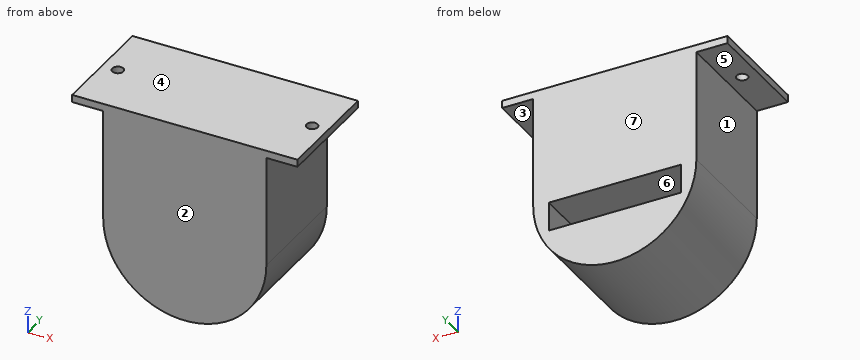
Autodesk Inventor part; units mm, degrees
ref_plane "YZ Plane" through (0, 0, 0) normal (1, 0, 0) x (0, 1, 0)
ref_plane "XZ Plane" through (0, 0, 0) normal (0, 1, 0) x (-1, 0, 0)
ref_plane "XY Plane" through (0, 0, 0) normal (0, 0, 1) x (1, 0, 0)
sketch "Sketch1" plane through (0, 0, 0) normal (0, 1, 0) x (-1, 0, 0)
  line L0 (-22, -14.1429) -> (-22, 15.8571)
  line L1 (-20.3963, 17.8571) -> (20.3963, 17.8571)
  line L2 (22, 15.8571) -> (22, -14.1429)
  arc A0 (-22, -14.1429) -> (22, -14.1429) centre (0, -14.1429) ccw
  line L3 (20.3963, 17.8571) -> (30.3963, 17.8571)
  line L4 (30.3963, 17.8571) -> (30.3963, 15.8571)
  line L5 (30.3963, 15.8571) -> (22, 15.8571)
  line L6 (-20.3963, 17.8571) -> (-30.3963, 17.8571)
  line L7 (-30.3963, 17.8571) -> (-30.3963, 15.8571)
  line L8 (-30.3963, 15.8571) -> (-22, 15.8571)
  point P0 (0, 0)
  point P1 (0, 17.8571)
  point P2 (22, 0)
  dimension "d1" = 2
  dimension "d2" = 2
  dimension "d3" = 10
  dimension "d4" = 10
  dimension "d5" = 30
  dimension "d6" = 22
extrude "Extrusion1" add sketch "Sketch1" along normal mid plane 30
sketch "Sketch2" plane through (0, 15, 0) normal (0, 1, 0) x (1, 0, 0)
  arc A0 (22, 14.1429) -> (-22, 14.1429) centre (0, 14.1429) ccw
  line L0 (-17.8, 22.1429) -> (17.8, 22.1429)
  line L1 (17.8, 22.1429) -> (17.8, 14.3429)
  line L2 (17.8, 14.3429) -> (-17.8, 14.3429)
  line L3 (-17.8, 14.3429) -> (-17.8, 22.1429)
  line L4 (-30.3963, -17.8571) -> (30.3963, -17.8571)
  point P0 (0, 0)
  point P1 (0, 36.1429)
  point P2 (0, 22.1429)
  dimension "d33" = 40
  dimension "d34" = 35.6
  dimension "d35" = 7.8
extrude "Extrusion2" cut sketch "Sketch2" against normal blind 25
sketch "Sketch3" plane through (30.3963, 15, 15.8571) normal (0, 0, -1) x (-1, 0, 0)
  line L0 (0, -30) -> (0, 0)
  line L1 (0, 0) -> (8.3963, 0)
  point P0 (30.3963, -15)
  point P1 (4.1982, -15)
  point P2 (0, -15)
  point P3 (4.1982, 0)
hole "Hole1" at (26.1982, 0, 15.8571) direction (0, 0, 1) diameter 3 depth 2
mirror "Mirror1" about plane through (0, 0, 0) normal (1, 0, 0) of "Hole1"
properties part number "Part_B7"
The listing builds one solid part. Answer for the finished solid, in the listing's coordinates (mm). Face numbers are marked on the shaded views. A direction names the side the tool comes from. Coordinates: 2 decimals unless noted, no trailing zeros. Loops run counter-clockwise (first coordinate to the right, second up) from the corner with the lowest first, then second, coordinate; pieces in that order, holes last. Notation, with made-up numbers: (-1, -14.5) -> (42, -14.5) arc R28 cw to (42, 6.5) -> close; hole circle Ø11 at (0.5, 15.5). An arc over 180 degrees is marked (long way). Answer in a Markdown table with one row per item. Add a question column.
1. The part is cut by section D-D, the plane z = 4. Write down the section's boundary in (x, y).
2. The part is cut by section B-B, the plane y = -7.75. Write down the section's boundary in (x, z), then the cut area to 3 significant figures.
3. Flat-ended cylindrical pins translate along their axes: P1, Ø4, axis at x = 8, y = 6, coming from the -Z side; P2, Ø4, axis at y = 3, z = -17, coming from the -X side; P3, Ø4, axis at x = 27, y = 2, coming from the -Z side; P4, Ø4, axis at x = -26.2, y = 0, coming from the +Z side. Find the tip coordinate at first contact, or state that the pin passes through.
4. For the marked faces 1, 2 and 3, determine the directions among +Z, -Z, +X, -X, +Y, -Y from which every point of the face is accessible in a straight line to the end or side of a thin tool.
5. Consider line 1 (X direction, y = 0, z = 16.75); line 2 (X direction, y = -9, z = 1); line 3 (X direction, y = 4, z = -20). Determine where each line is inside the solid, lowest interval first. Write a range as [from, to].
6. Determine the mould class of the marked faces 4, 5, 6 and 7 for opening direction Z: +Z half, -Z half, draft (parallel to the pull), parting line (faces both ways), or undercut.
7. The part is cut by section C-C, the plane x = 0. Write down the section's boundary in (y, z), then the cut area to 4 significant figures.
8. The part is cut by section A-A, the plane y = 0. Write down the section's boundary in (x, z).
Answer below:
| question | item | result |
|---|---|---|
| 1 | outline | (-22, -15) -> (22, -15) -> (22, 15) -> (-22, 15) -> close |
| 2 | outline | (-30.4, 15.86) -> (-22, 15.86) -> (-22, -14.14) arc R22 ccw to (22, -14.14) -> (22, 15.86) -> (30.4, 15.86) -> (30.4, 17.86) -> (-30.4, 17.86) -> close; hole (-17.8, -22.14) -> (17.8, -22.14) -> (17.8, -14.34) -> (-17.8, -14.34) -> close |
| 2 | area | 1,920 mm2 |
| 3 | P1 | z = -35.31 |
| 3 | P2 | x = -21.98 |
| 3 | P3 | z = 15.86 |
| 3 | P4 | z = 17.86 |
| 4 | face 1 | -Z, -X, +Y, -Y |
| 4 | face 2 | +Z, -Z, +X, -X, -Y |
| 4 | face 3 | -Z, +X, +Y, -Y |
| 5 | line 1 | [-30.4, -27.7], [-24.7, 24.7], [27.7, 30.4] |
| 5 | line 2 | [-22, 22] |
| 5 | line 3 | [-21.21, -17.8], [17.8, 21.21] |
| 6 | face 4 | +Z half |
| 6 | face 5 | -Z half |
| 6 | face 6 | undercut |
| 6 | face 7 | draft |
| 7 | outline | (-15, -36.14) -> (15, -36.14) -> (15, -22.14) -> (-10, -22.14) -> (-10, -14.34) -> (15, -14.34) -> (15, 17.86) -> (-15, 17.86) -> close |
| 7 | area | 1,425 mm2 |
| 8 | outline | (-30.4, 15.86) -> (-27.7, 15.86) -> (-27.7, 17.86) -> (-30.4, 17.86) -> close; (-24.7, 15.86) -> (-22, 15.86) -> (-22, -14.14) arc R22 ccw to (22, -14.14) -> (22, 15.86) -> (24.7, 15.86) -> (24.7, 17.86) -> (-24.7, 17.86) -> close; (27.7, 15.86) -> (30.4, 15.86) -> (30.4, 17.86) -> (27.7, 17.86) -> close; hole (-17.8, -22.14) -> (17.8, -22.14) -> (17.8, -14.34) -> (-17.8, -14.34) -> close |
